Part model, mm, in its own coordinate system. Round coordinates to 2 decimals unless told otherwise and drop trailing zeros. Write each loop counter-clockwise with the first axis right and the second up, starting at its lowest first coordinate (ties: lowest second). Pieces come first, ordered by that corner, then holes. Notation, with made-up numbers: M 7.25,28 L 37.25,28 A16 ccw 37.25,47 Z; hole C 74.25,-36 d7. An arc over 180 degrees is marked long. Use a Markdown table: item, result. Add a question column.
1) Slice it at A-A on x = -204. Write the cut outline in (y, z), plus the area to 3 significant figures.
2) Slice it at B-B on y = 60. Write the cut outline in (x, z).
3) Drop flat-ended pins along their axis: P1, Ø1.5, axis at x = -154.5, z = 1, coming from the +Y side; P2, Ø1.5, axis at x = -210, z = 1.5, coming from the +Y side; P3, Ø0.9, axis at y = 44, z = 1.5, coming from the -X side. Give the stop position or say it passes through.
4) Slice it at D-D on y = 33. Write the cut outline in (x, z), plus the area to 3 significant figures.
5) Slice it at C-C on z = 0.6. Give the number of separate pieces and of enclosed holes in the cut face, plus the area to 3 significant figures.
6) Wall check: probe 1 along X at (y, z) = (48, 0.3); probe 2 along X at (y, z) = (114, 2.85); probe 3 along Y at (x, z) = (-149, 0.2). Give the ranges that are in metal, low to high.
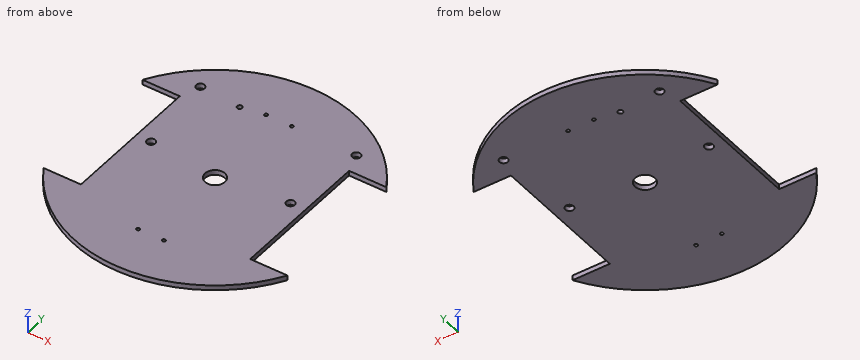
```python
from build123d import *

# Parameters (mm, degrees)
ESQUISSE1_R              = 85
BOSS_EXTRU_1_DEPTH       = 3
ESQUISSE2_W              = 32.5
ESQUISSE2_H              = 85
ENL_V_MAT_EXTRU_6_DEPTH  = 3
ESQUISSE3_R              = 1
ENL_V_MAT_EXTRU_8_DEPTH  = 10
ESQUISSE53_R             = 2.5
ENL_V_MAT_EXTRU_21_DEPTH = 10
ESQUISSE54_R             = 2.5
ENL_V_MAT_EXTRU_22_DEPTH = 10
ESQUISSE55_R             = 1.5
ENL_V_MAT_EXTRU_23_DEPTH = 10
ESQUISSE56_R             = 6
ENL_V_MAT_EXTRU_24_DEPTH = 10


with BuildPart() as part:
    # Esquisse1 → Boss.-Extru.1 (new body)
    with BuildSketch(Plane.XY):
        with Locations((-147.95974357, 62.548931244)):
            Circle(ESQUISSE1_R)
    extrude(amount=BOSS_EXTRU_1_DEPTH)

    # Esquisse2 → Enlèv. mat.-Extru.6 (cut)
    with BuildSketch(Plane.XY):
        with BuildLine():
            Line((-199.071902892, 105.048931244), (-221.571902892, 105.048931244))
            ThreePointArc((-221.571902892, 105.048931244), (-227.739869981, 91.876928617), (-231.571902892, 77.846212492))
            Line((-231.571902892, 77.846212492), (-231.571902892, 47.251649997))
            ThreePointArc((-231.571902892, 47.251649997), (-227.739869981, 33.220933871), (-221.571902892, 20.048931244))
            Line((-221.571902892, 20.048931244), (-199.071902892, 20.048931244))
            Line((-199.071902892, 20.048931244), (-199.071902892, 105.048931244))
        make_face()
        with Locations((-80.597584249, 62.548931244)):
            Rectangle(ESQUISSE2_W, ESQUISSE2_H)
    extrude(amount=ENL_V_MAT_EXTRU_6_DEPTH, mode=Mode.SUBTRACT)


with BuildPart() as enl_v_mat_extru_6_piece_1:
    # of the separate pieces the step leaves, piece 1, a body of its own (enl_v_mat_extru_6_pieces)
    add(part.part.solids().sort_by_distance((-74.347584249, 105.048931244, 0))[0])

    # Esquisse3 → Enlèv. mat.-Extru.8 (cut)
    with BuildSketch(Plane.XY.offset(3)):
        with Locations((-155.70974357, 117.548931244)):
            Circle(ESQUISSE3_R)
        with Locations((-140.20974357, 117.548931244)):
            Circle(ESQUISSE3_R)
        with Locations((-140.20974357, 7.548931244)):
            Circle(ESQUISSE3_R)
        with Locations((-155.70974357, 7.548931244)):
            Circle(ESQUISSE3_R)
    extrude(amount=-ENL_V_MAT_EXTRU_8_DEPTH, mode=Mode.SUBTRACT)

    # Esquisse53 → Enlèv. mat.-Extru.21 (cut)
    with BuildSketch(Plane(origin=(0, 0, 0), x_dir=(-1, 0, 0), z_dir=(0, 0, -1))):
        with Locations((190.071902892, 67.548931244)):
            Circle(ESQUISSE53_R)
        with Locations((105.847584249, 67.548931244)):
            Circle(ESQUISSE53_R)
    extrude(amount=-ENL_V_MAT_EXTRU_21_DEPTH, mode=Mode.SUBTRACT)

    # Esquisse54 → Enlèv. mat.-Extru.22 (cut)
    with BuildSketch(Plane(origin=(0, 0, 0), x_dir=(-1, 0, 0), z_dir=(0, 0, -1))):
        with Locations((195.071902892, 117.048931244)):
            Circle(ESQUISSE54_R)
        with Locations(Location((100.847584249, 117.048931244, 0), (0, 0, 180))):
            Circle(ESQUISSE54_R)
    extrude(amount=-ENL_V_MAT_EXTRU_22_DEPTH, mode=Mode.SUBTRACT)

    # Esquisse55 → Enlèv. mat.-Extru.23 (cut)
    with BuildSketch(Plane(origin=(0, 0, 0), x_dir=(-1, 0, 0), z_dir=(0, 0, -1))):
        with Locations((169.95974357, 115.048931244)):
            Circle(ESQUISSE55_R)
    extrude(amount=-ENL_V_MAT_EXTRU_23_DEPTH, mode=Mode.SUBTRACT)

    # Esquisse56 → Enlèv. mat.-Extru.24 (cut)
    with BuildSketch(Plane(origin=(0, 0, 0), x_dir=(-1, 0, 0), z_dir=(0, 0, -1))):
        with Locations((147.95974357, 62.548931244)):
            Circle(ESQUISSE56_R)
    extrude(amount=-ENL_V_MAT_EXTRU_24_DEPTH, mode=Mode.SUBTRACT)


with BuildPart() as enl_v_mat_extru_6_piece_2:
    # of the separate pieces the step leaves, piece 2, a body of its own (enl_v_mat_extru_6_pieces)
    add(part.part.solids().sort_by_distance((-64.347584249, 47.251649997, 0))[0])


with BuildPart() as enl_v_mat_extru_6_piece_3:
    # of the separate pieces the step leaves, piece 3, a body of its own (enl_v_mat_extru_6_pieces)
    add(part.part.solids().sort_by_distance((-231.571902892, 77.846212492, 0))[0])


solid = enl_v_mat_extru_6_piece_1.part
```
Entries:
| question | item | result |
|---|---|---|
| 1 | outline | M -1.36,0 L 20.05,0 L 20.05,3 L -1.36,3 Z; M 105.05,0 L 126.46,0 L 126.46,3 L 105.05,3 Z |
| 1 | area | 128 mm^2 |
| 2 | outline | M -199.07,0 L -153.39,0 L -153.39,3 L -199.07,3 Z; M -142.53,0 L -96.85,0 L -96.85,3 L -142.53,3 Z |
| 3 | P1 | stops at y = 147.35 |
| 3 | P2 | stops at y = 121.44 |
| 3 | P3 | stops at x = -199.07 |
| 4 | outline | M -199.07,0 L -96.85,0 L -96.85,3 L -199.07,3 Z |
| 4 | area | 307 mm^2 |
| 5 | separate pieces | 1 |
| 5 | enclosed holes | 10 |
| 5 | area | 17,400 mm^2 |
| 6 | probe 1 | x = -199.07 to -96.85 |
| 6 | probe 2 | x = -215.62 to -171.03, -168.89 to -80.3 |
| 6 | probe 3 | y = -22.44 to 56.64, 68.46 to 147.54 |
